Drawing for the job (mm, zero at the part's lowest x, y, z). A direction names the side the tool comes from. Give positions to 0.01 mm unless a question says otherwise; leave off trailing zeros. Loops run counter-clockwise (first coordinate to the right, second up) from the corner with the lowest first, then second, coordinate; pieces in that order, holes last. Notation, with made-up numbers: M -14.5,31 L 40.5,31 A25 cw 40.5,45 Z; hole C -29.75,57.5 d10. An arc over 180 degrees is marked long. Use CSV: the item, a comma, the result in double quotes. Start each with the question number.
(1) Slice it at D-D on x = 0.75. List the corners of the cut face in (y, z), and give its area (3 significant figures).
(2) Flat gauge pins, fed straight in: P1, Ø3, axis at x = 5, y = 31.5, coming from the +Z side; P2, Ø2, axis at x = 5, y = 7.5, coming from the +Z side. Where does each tip first touch, or does it go through?
(3) Slice it at A-A on y = 46.5. List the corners of the cut face in (x, z).
(4) Tool access for the marked faces 1 and 2: list every direction of +Z, -Z, +X, -X, +Y, -Y with a clear straight run to the whole face (end or side of a thin tool).
(5) Slice it at B-B on z = 5.5. List the corners of the cut face in (x, y), and give its area (3 significant figures).
(6) Wall check: line 1 along Y through (x, z) = (5, 4.75); line 2 along Y through (x, z) = (5, 1.75); line 3 along Y through (x, z) = (8, 3.5). Give the ranges that are in metal, low to high. Write a range as from..to.
(7) Slice it at C-C on x = 5. List the corners of the cut face in (y, z).
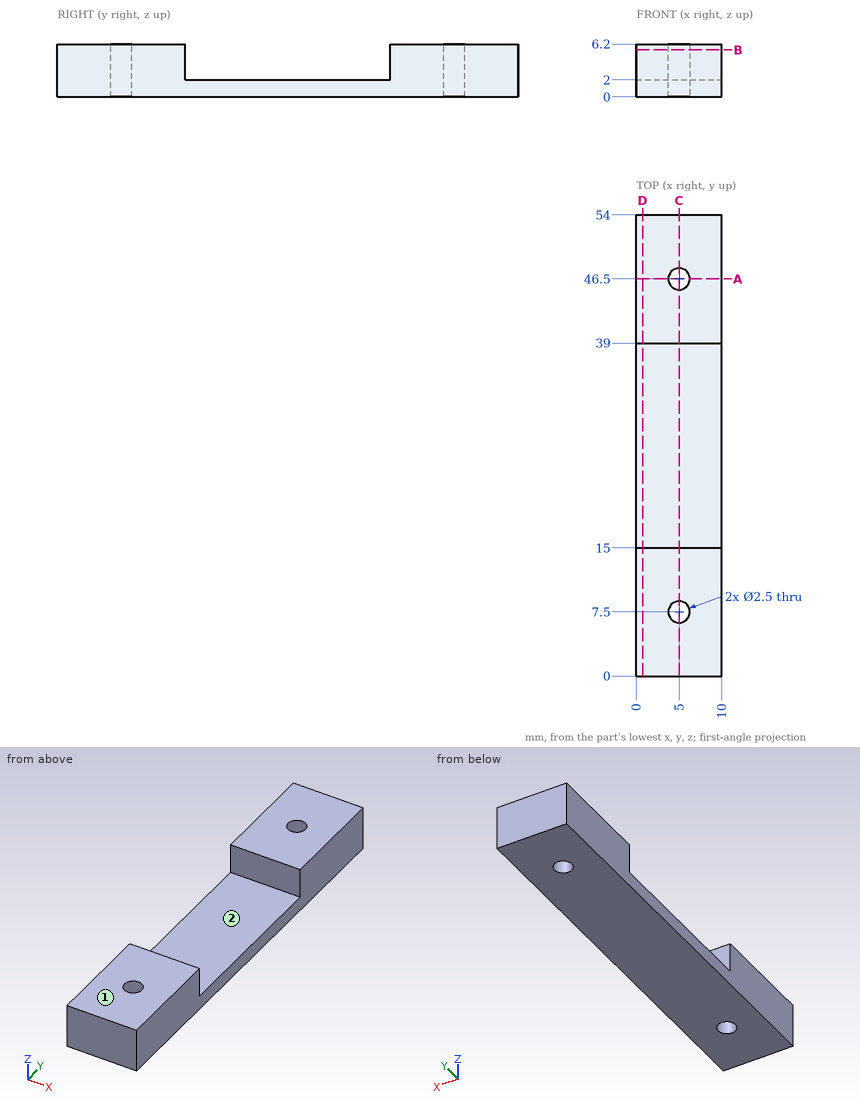
Reply:
1,outline,"M 0,0 L 54,0 L 54,6.2 L 39,6.2 L 39,2 L 15,2 L 15,6.2 L 0,6.2 Z"
1,area,"234 mm^2"
2,P1,"stops at z = 2"
2,P2,"passes through"
3,outline,"M 0,0 L 3.75,0 L 3.75,6.2 L 0,6.2 Z; M 6.25,0 L 10,0 L 10,6.2 L 6.25,6.2 Z"
4,face 1,"+Z, +X, -X, +Y, -Y"
4,face 2,"+Z, +X, -X"
5,outline,"M 0,0 L 10,0 L 10,15 L 0,15 Z; M 0,39 L 10,39 L 10,54 L 0,54 Z; hole C 5,7.5 d2.5; hole C 5,46.5 d2.5"
5,area,"290 mm^2"
6,line 1,"y = 0..6.25, 8.75..15, 39..45.25, 47.75..54"
6,line 2,"y = 0..6.25, 8.75..45.25, 47.75..54"
6,line 3,"y = 0..15, 39..54"
7,outline,"M 0,0 L 6.25,0 L 6.25,6.2 L 0,6.2 Z; M 8.75,0 L 45.25,0 L 45.25,6.2 L 39,6.2 L 39,2 L 15,2 L 15,6.2 L 8.75,6.2 Z; M 47.75,0 L 54,0 L 54,6.2 L 47.75,6.2 Z"
